```python
from build123d import *

# Parameters (mm, degrees)
SKETCH_1_W          = 131.5
SKETCH_1_H          = 3.6
EXTRUDE_1_DEPTH     = 4
SKETCH_2_W          = 4
SKETCH_2_H          = 3.6
EXTRUDE_2_DEPTH     = 28
SKETCH_3_W          = 4
SKETCH_3_H          = 3.6
EXTRUDE_3_DEPTH     = 28
SKETCH_4_W          = 4
SKETCH_4_H          = 3.6
EXTRUDE_4_DEPTH     = 123.5
SKETCH_5_W          = 8
SKETCH_5_H          = 32
EXTRUDE_5_DEPTH     = 8
CUT_EXTRUDE_1_REACH = 137.574
SKETCH_6_R          = 3
EXTRUDE_6_REACH     = 136.686
SKETCH_7_W          = 25
SKETCH_7_H          = 3.6
EXTRUDE_7_REACH     = 109.677
SKETCH_8_W          = 3.6
SKETCH_8_H          = 3.6
SKETCH_13_W         = 10
SKETCH_13_H         = 10
EXTRUDE_8_DEPTH     = 10
EXTRUDE_9_REACH     = 136.019
SKETCH_14_W         = 12
SKETCH_14_H         = 3.6
SKETCH_15_W         = 6
SKETCH_15_H         = 13.6
EXTRUDE_10_DEPTH    = 10
EXTRUDE_11_REACH    = 114.032
SKETCH_16_R         = 3
SKETCH_17_W         = 100.5
SKETCH_17_H         = 2
EXTRUDE_12_DEPTH    = 2
SKETCH_18_W         = 100.5
SKETCH_18_H         = 1.6
EXTRUDE_13_DEPTH    = 2


with BuildPart() as part:
    # 草图1 → 凸台-拉伸1 (new body)
    with BuildSketch(Plane.XY):
        with Locations((65.75, 1.8)):
            Rectangle(SKETCH_1_W, SKETCH_1_H)
    extrude(amount=-EXTRUDE_1_DEPTH)

    # 草图2 → 凸台-拉伸2 (add)
    with BuildSketch(Plane(origin=(0, 0, -4), x_dir=(-1, 0, 0), z_dir=(0, 0, -1))):
        with Locations((-2, 1.8)):
            Rectangle(SKETCH_2_W, SKETCH_2_H)
    extrude(amount=EXTRUDE_2_DEPTH)

    # 草图3 → 凸台-拉伸3 (add)
    with BuildSketch(Plane(origin=(0, 0, -4), x_dir=(-1, 0, 0), z_dir=(0, 0, -1))):
        with Locations((-129.5, 1.8)):
            Rectangle(SKETCH_3_W, SKETCH_3_H)
    extrude(amount=EXTRUDE_3_DEPTH)

    # 草图4 → 凸台-拉伸4 (add)
    with BuildSketch(Plane(origin=(4, 0, 0), x_dir=(0, 0, -1), z_dir=(1, 0, 0))):
        with Locations((30, 1.8)):
            Rectangle(SKETCH_4_W, SKETCH_4_H)
    extrude(amount=EXTRUDE_4_DEPTH)

    # 草图5 → 凸台-拉伸5 (add)
    with BuildSketch(Plane.XZ):
        with Locations((118.5, -16)):
            Rectangle(SKETCH_5_W, SKETCH_5_H)
    extrude(amount=EXTRUDE_5_DEPTH)

    # 草图6 → 切除-拉伸1 (cut, up to next)
    with BuildSketch(Plane.XY, mode=Mode.PRIVATE) as cut_extrude_1_sk1:
        with Locations((118.5, -4)):
            Circle(SKETCH_6_R)
    cut_extrude_1_tool1 = extrude(cut_extrude_1_sk1.sketch, amount=-CUT_EXTRUDE_1_REACH, mode=Mode.PRIVATE) & part.part
    add(cut_extrude_1_tool1.solids().sort_by_distance((118.5, -4, 0))[0], mode=Mode.SUBTRACT)

    # 草图7 → 凸台-拉伸6 (add, up to next)
    with BuildSketch(Plane(origin=(0, 0, -4), x_dir=(-1, 0, 0), z_dir=(0, 0, -1)), mode=Mode.PRIVATE) as extrude_6_sk1:
        with Locations((-115, 1.8)):
            Rectangle(SKETCH_7_W, SKETCH_7_H)
    extrude_6_tool1 = extrude(extrude_6_sk1.sketch, amount=EXTRUDE_6_REACH, mode=Mode.PRIVATE) - part.part
    add(extrude_6_tool1.solids().sort_by_distance((115, 1.8, -4))[0])

    # 草图8 → 凸台-拉伸7 (add, up to next)
    with BuildSketch(Plane.ZY.offset(-102.5), mode=Mode.PRIVATE) as extrude_7_sk1:
        with Locations((-11.8, 1.8)):
            Rectangle(SKETCH_8_W, SKETCH_8_H)
    extrude_7_tool1 = extrude(extrude_7_sk1.sketch, amount=EXTRUDE_7_REACH, mode=Mode.PRIVATE) - part.part
    add(extrude_7_tool1.solids().sort_by_distance((102.5, 1.8, -11.8))[0])

    # 草图13 → 凸台-拉伸8 (add)
    with BuildSketch(Plane(origin=(0, 3.6, 0), x_dir=(1, 0, 0), z_dir=(0, 1, 0))):
        with Locations((111.5, 7)):
            Rectangle(SKETCH_13_W, SKETCH_13_H)
    extrude(amount=EXTRUDE_8_DEPTH)

    # 草图14 → 凸台-拉伸9 (add, up to next)
    with BuildSketch(Plane.XY.offset(-10), mode=Mode.PRIVATE) as extrude_9_sk1:
        with Locations((10, 1.8)):
            Rectangle(SKETCH_14_W, SKETCH_14_H)
    extrude_9_tool1 = extrude(extrude_9_sk1.sketch, amount=EXTRUDE_9_REACH, mode=Mode.PRIVATE) - part.part
    add(extrude_9_tool1.solids().sort_by_distance((10, 1.8, -10))[0])

    # 草图15 → 凸台-拉伸10 (add)
    with BuildSketch(Plane(origin=(0, 3.6, 0), x_dir=(1, 0, 0), z_dir=(0, 1, 0))):
        with Locations((13, 6.8)):
            Rectangle(SKETCH_15_W, SKETCH_15_H)
    extrude(amount=EXTRUDE_10_DEPTH)

    # 草图16 → 凸台-拉伸11 (add, up to next)
    with BuildSketch(Plane.ZY.offset(-106.5), mode=Mode.PRIVATE) as extrude_11_sk1:
        with Locations(Location((-7, 8.6, 0), (0, 0, 180))):
            Circle(SKETCH_16_R)
    extrude_11_tool1 = extrude(extrude_11_sk1.sketch, amount=EXTRUDE_11_REACH, mode=Mode.PRIVATE) - part.part
    add(extrude_11_tool1.solids().sort_by_distance((106.5, 8.6, -7))[0])

    # 草图17 → 凸台-拉伸12 (add)
    with BuildSketch(Plane(origin=(0, 3.6, 0), x_dir=(1, 0, 0), z_dir=(0, 1, 0))):
        with Locations((66.25, 1)):
            Rectangle(SKETCH_17_W, SKETCH_17_H)
    extrude(amount=EXTRUDE_12_DEPTH)

    # 草图18 → 凸台-拉伸13 (add)
    with BuildSketch(Plane(origin=(0, 3.6, 0), x_dir=(1, 0, 0), z_dir=(0, 1, 0))):
        with Locations((66.25, 12.8)):
            Rectangle(SKETCH_18_W, SKETCH_18_H)
    extrude(amount=EXTRUDE_13_DEPTH)


solid = part.part
```
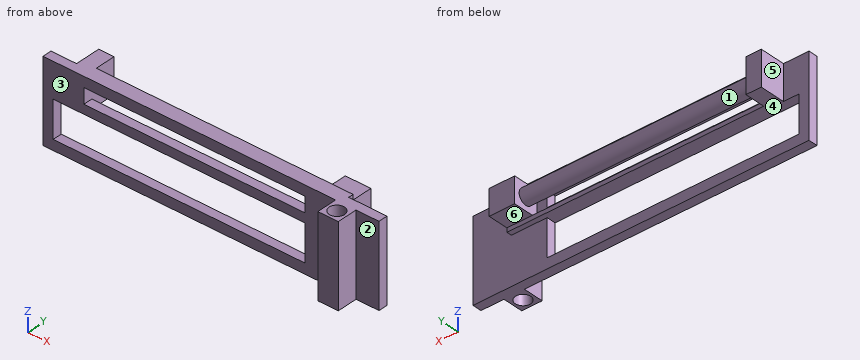
Part model, mm, in its own coordinate system. Face numbers are marked on the shaded views. A direction names the side the tool comes from. Round coordinates to 2 decimals unless told otherwise and drop trailing zeros. Write each loop counter-clockwise with the first axis right and the second up, starting at its lowest first coordinate (ties: lowest second). Pieces come first, ordered by that corner, then holes. Notation, with made-up numbers: (-15.5, -1.75) -> (16.5, -1.75) arc R25 ccw to (16.5, 18.25) -> close; hole circle Ø3 at (78.25, 84.5). An arc over 180 degrees is marked (long way). Return JSON: item names as keys, results as strings. Group by question number.
Q1. Probe L1, parallel to Z at x = 77, y = 3.5; L2, parallel to X at y = 1.5, z = -22.5; L3, parallel to Z at x = 95.5, y = 5.25. List the from-to ranges inside material, lowest first. Write a range as [from, to].
Q2. Saw through at C-C on z = -7. Write the cut outline in (x, y).
Q3. Which spindle directions (+Z, -Z, +X, -X, +Y, -Y) get a long thin tool onto all of the face, cutting with end or side? Do the marked faces 1, 2 and 3. Say none if no direction does.
Q4. Saw through at A-A on y = -4. Write the cut outline in (x, z).
Q5. Pin check, flat tips, straight feed: pin 1 (1 mm diameter, centred on y = -2.5, z = -20.5, fed in from -X); pin 2 (10 mm diameter, centred on x = 62.5, y = 10.5, fed in from -Z); pin 3 (3 mm diameter, centred on y = 11.5, z = -6, fed in from +X). Stop position of each tip, or through.
Q6. Saw through at D-D on y = 1.5. Write the cut outline in (x, z), plus the area to 3 significant figures.
Q7. Saw through at B-B on z = -17.5. Write the cut outline in (x, y).
Q8. Mould opens along X. For the marked faces 4, 5 and 6 say: pulls with the +X half, pulls with the -X half, needs draft (parallel to the pull), parting line crosses it, or undercut.
Answer:
{
 "1": {"L1": "[-32, -28], [-13.6, -10], [-4, 0]", "L2": "[0, 4], [102.5, 131.5]", "L3": "[-13.6, -12], [-2, 0]"},
 "2": {"outline": "(0, 0) -> (16, 0) -> (16, 5.6) -> (106.5, 5.6) -> (106.5, 3.6) -> (102.5, 3.6) -> (102.5, 0) -> (114.5, 0) -> (114.5, -8) -> (122.5, -8) -> (122.5, 0) -> (131.5, 0) -> (131.5, 3.6) -> (116.5, 3.6) -> (116.5, 13.6) -> (106.5, 13.6) -> (106.5, 11.6) -> (16, 11.6) -> (16, 13.6) -> (10, 13.6) -> (10, 3.6) -> (0, 3.6) -> close; hole circle Ø6 at (118.5, -4)"},
 "3": {"face 1": "none", "face 2": "+Z, -Z, +X, -Y", "face 3": "+Z, -Z, -X, -Y"},
 "4": {"outline": "(114.5, -32) -> (115.5, -32) -> (115.5, 0) -> (114.5, 0) -> close; (121.5, -32) -> (122.5, -32) -> (122.5, 0) -> (121.5, 0) -> close"},
 "5": {"pin 1": "x = 114.5", "pin 2": "z = -13.6", "pin 3": "x = 116.5"},
 "6": {"outline": "(0, -32) -> (131.5, -32) -> (131.5, 0) -> (0, 0) -> close; hole (4, -28) -> (102.5, -28) -> (102.5, -13.6) -> (4, -13.6) -> close; hole (16, -10) -> (102.5, -10) -> (102.5, -4) -> (16, -4) -> close", "area": "2,270 mm2"},
 "7": {"outline": "(0, 0) -> (4, 0) -> (4, 3.6) -> (0, 3.6) -> close; (102.5, 0) -> (114.5, 0) -> (114.5, -8) -> (122.5, -8) -> (122.5, 0) -> (131.5, 0) -> (131.5, 3.6) -> (102.5, 3.6) -> close; hole circle Ø6 at (118.5, -4)"},
 "8": {"face 4": "undercut", "face 5": "pulls with the -X half", "face 6": "needs draft"}
}
